from build123d import *

# Parameters (mm, degrees)
BOX017_W                    = 12.6
BOX017_H                    = 10
BOX017_DEPTH                = 2
BOX016_W                    = 3
BOX016_H                    = 6
BOX016_DEPTH                = 20
BOX015_W                    = 3
BOX015_H                    = 6
BOX015_DEPTH                = 20
BOX013_W                    = 12.6
BOX013_H                    = 10
BOX013_DEPTH                = 1
CYLINDER016_R               = 4.5
CYLINDER016_DEPTH           = 1.5
SKETCH018_R                 = 2.1
PAD011_DEPTH                = 0.8
CYLINDER015_R               = 14
CYLINDER015_DEPTH           = 19
CYLINDER018_W               = 16
CYLINDER018_H               = 14
CYLINDER018_ANGLE           = 80
CYLINDER018_PLACEMENT_ANGLE = 230
BOX014_W                    = 14.6
BOX014_H                    = 5
BOX014_DEPTH                = 16.2
POCKET002_DEPTH             = 0.6
PAD012_DEPTH                = 1.5


with BuildPart() as cubo013:
    # Box017 → Box017 (new body)
    with BuildSketch(Plane(origin=(-6.3, -16, 18), x_dir=(1, 0, 0), z_dir=(0, 0, 1))):
        with Locations((6.3, 5)):
            Rectangle(BOX017_W, BOX017_H)
    extrude(amount=BOX017_DEPTH)


with BuildPart() as cubo012:
    # Box016 → Box016 (new body)
    with BuildSketch(Plane(origin=(-12, -15, 0), x_dir=(1, 0, 0), z_dir=(0, 0, 1))):
        with Locations((1.5, 3)):
            Rectangle(BOX016_W, BOX016_H)
    extrude(amount=BOX016_DEPTH)


with BuildPart() as obj1:
    # Box015 → Box015 (new body)
    with BuildSketch(Plane(origin=(9, -15, 0), x_dir=(1, 0, 0), z_dir=(0, 0, 1))):
        with Locations((1.5, 3)):
            Rectangle(BOX015_W, BOX015_H)
    extrude(amount=BOX015_DEPTH)

    # Fusion011: union Cubo012
    add(cubo012.part)


with BuildPart() as cubo009:
    # Box013 → Box013 (new body)
    with BuildSketch(Plane(origin=(-6.3, -16, 18), x_dir=(1, 0, 0), z_dir=(0, 0, 1))):
        with Locations((6.3, 5)):
            Rectangle(BOX013_W, BOX013_H)
    extrude(amount=BOX013_DEPTH)


with BuildPart() as cilindro008:
    # Cylinder016 → Cylinder016 (new body)
    with BuildSketch(Plane(origin=(0, 8, 19), x_dir=(1, 0, 0), z_dir=(0, 0, 1))):
        Circle(CYLINDER016_R)
    extrude(amount=CYLINDER016_DEPTH)


with BuildPart() as pad011:
    # Sketch018 → Pad011 (new body)
    with BuildSketch(Plane.XY.offset(18.2)):
        with BuildLine():
            ThreePointArc((-17.5, 3.5), (-21, 0), (-17.5, -3.5))
            Line((-17.5, -3.5), (17.5, -3.5))
            ThreePointArc((17.5, -3.5), (21, 0), (17.5, 3.5))
            Line((-17.5, 3.5), (17.5, 3.5))
        make_face()
        with Locations((-17.5, 0)):
            Circle(SKETCH018_R, mode=Mode.SUBTRACT)
        with Locations((17.5, 0)):
            Circle(SKETCH018_R, mode=Mode.SUBTRACT)
    extrude(amount=PAD011_DEPTH)


with BuildPart() as body001:
    # Cylinder015 → Cylinder015 (new body)
    with BuildSketch(Plane.XY):
        Circle(CYLINDER015_R)
    extrude(amount=CYLINDER015_DEPTH)

    # Fusion007: union Pad011
    add(pad011.part)

    # Fusion009: union Cilindro008
    add(cilindro008.part)

    # Fusion010: union Cubo009
    add(cubo009.part)


with BuildPart() as cut021:
    # Cylinder018 → Cylinder018 (revolve)
    with BuildSketch(Plane.XZ):
        with Locations((8, 7)):
            Rectangle(CYLINDER018_W, CYLINDER018_H)
    revolve(axis=Axis((0, 0, 0), (0, 0, 1)), revolution_arc=CYLINDER018_ANGLE)


with BuildPart() as cut021_1:
    # Cylinder018 placement: moved
    add(cut021.part.moved(Location((0, 0, 3))).rotate(Axis((0, 0, 3), (0, 0, 1)), CYLINDER018_PLACEMENT_ANGLE))

    # Cut020: cut Body001
    add(body001.part, mode=Mode.SUBTRACT)

    # Cut021: cut obj1
    add(obj1.part, mode=Mode.SUBTRACT)


with BuildPart() as plastic_base_final001:
    # Box014 → Box014 (new body)
    with BuildSketch(Plane(origin=(-7.3, -17, 3), x_dir=(1, 0, 0), z_dir=(0, 0, 1))):
        with Locations((7.3, 2.5)):
            Rectangle(BOX014_W, BOX014_H)
    extrude(amount=BOX014_DEPTH)

    # Cut019: cut Body001
    add(body001.part, mode=Mode.SUBTRACT)

    # Fusion012: union Cut021
    add(cut021_1.part)

    # Cut022: cut Cubo013
    add(cubo013.part, mode=Mode.SUBTRACT)

    # Sketch019 (on Face5 of Cut022) → Pocket002 (cut)
    with BuildSketch(Plane.XZ.offset(17)):
        with BuildLine():
            ThreePointArc((-4, 18.3), (-4.6, 17.7), (-4, 17.1))
            Line((-4, 17.1), (4, 17.1))
            ThreePointArc((4, 17.1), (4.6, 17.7), (4, 18.3))
            Line((-4, 18.3), (4, 18.3))
        make_face()
    extrude(amount=-POCKET002_DEPTH, mode=Mode.SUBTRACT)

    # Sketch020 (on Face17 of Pocket002) → Pad012 (new body)
    with BuildSketch(Plane(origin=(0, 0, 3), x_dir=(1, 0, 0), z_dir=(0, 0, -1))):
        with BuildLine():
            ThreePointArc((9, 11.496086), (0, 14.6), (-9, 11.496086))
            Line((-9, 11.496086), (-9, 10.723805))
            ThreePointArc((9, 10.723805), (0, 14), (-9, 10.723805))
            Line((9, 11.496086), (9, 10.723805))
        make_face()
    extrude(amount=PAD012_DEPTH)


solid = plastic_base_final001.part
Build history of the part. All positions in model axes, mm. A direction names the side the tool comes from. Round coordinates to 2 decimals unless told otherwise and drop trailing zeros. Loops run counter-clockwise (first coordinate to the right, second up) from the corner with the lowest first, then second, coordinate; pieces in that order, holes last. Notation, with made-up numbers: (72.5, 16) -> (128.5, 16) arc R16 cw to (128.5, 43) -> close; hole circle Ø6 at (31, -38). An arc over 180 degrees is marked (long way). Use CSV: the item, a comma, the result in double quotes. Start each with the question number.
Q1. Mould opens along X. For faces 1 (the face through (0, -17, 11)), 2 (the face through (-9, -12, 9)), 3 (the face through (0, -15, 18)), 4 (the face through (-6.3, -14, 19)) say: +X half, -X half, draft (parallel to the pull), parting line (faces both ways), or undercut.
Q2. Flat gauge pins, fed straight in: pin 1 Ø0.5 at (x, y) = (8.5, -13) entering from +Z; pin 2 Ø0.5 at (x, y) = (0.5, -17) entering from -Z; pin 3 Ø4 at (x, z) = (5.5, 14.5) entering from +Y; pin 4 Ø1.5 at (x, y) = (-1.5, -12) entering from +Z. Where does each tip first touch, or does it go through?
Q3. Drill centre lines: L1, parallel to Z at x = -2, y = -16.5; L2, parallel to Z at x = -6.75, y = -13.5; L3, parallel to X at y = -14.5, z = 7.25. Where is each one in solid material? Low to high.
Q4. Saw through at B-B on x = -3. Give the cut face in (y, z), and give its area (3 significant figures).
Q5. Which spindle directions (+Z, -Z, +X, -X, +Y, -Y) get a long thin tool onto all of the face, cutting with end or side? Do faces 5 (the face through (0, -15, 3)), 6 (the face through (0, -16.4, 18)), 7 (the face through (9, -12, 9)), 8 (the face through (0, -16, 19)). Say none if no direction does.
Solutions:
1,face 1,"draft"
1,face 2,"-X half"
1,face 3,"undercut"
1,face 4,"undercut"
2,pin 1,"stops at z = 17"
2,pin 2,"stops at z = 3"
2,pin 3,"stops at y = -11.82"
2,pin 4,"passes through"
3,L1,"z = 3 to 17.1, 18.3 to 19.2"
3,L2,"z = 3 to 19.2"
3,L3,"x = -7.3 to 7.3"
4,outline,"(-17, 3) -> (-14.29, 3) -> (-14.29, 1.5) -> (-13.67, 1.5) -> (-13.67, 18) -> (-16, 18) -> (-16, 19.2) -> (-17, 19.2) -> (-17, 18.3) -> (-16.4, 18.3) -> (-16.4, 17.1) -> (-17, 17.1) -> close"
4,area,"51.3 mm^2"
5,face 5,"-Z, -Y"
5,face 6,"-Y"
5,face 7,"+Z, -Z, +X, +Y, -Y"
5,face 8,"+Z, +Y"
